Can you work these out from the drawing? Everything is in mm from the part's minimum corner. Coordinates: 2 decimals unless noted, no trailing zeros. Write each loop counter-clockwise with the first axis right and the second up, starting at its lowest first coordinate (ties: lowest second). Pieces come first, ordered by that corner, then holes. Notation, with made-up numbers: M -18.5,65.5 L 18.5,65.5 A30 ccw 18.5,95.5 Z; hole C 11.5,32.25 d11. An arc over 180 degrees is marked long. Answer as a JSON object with one key per item and string values. Group by question number.
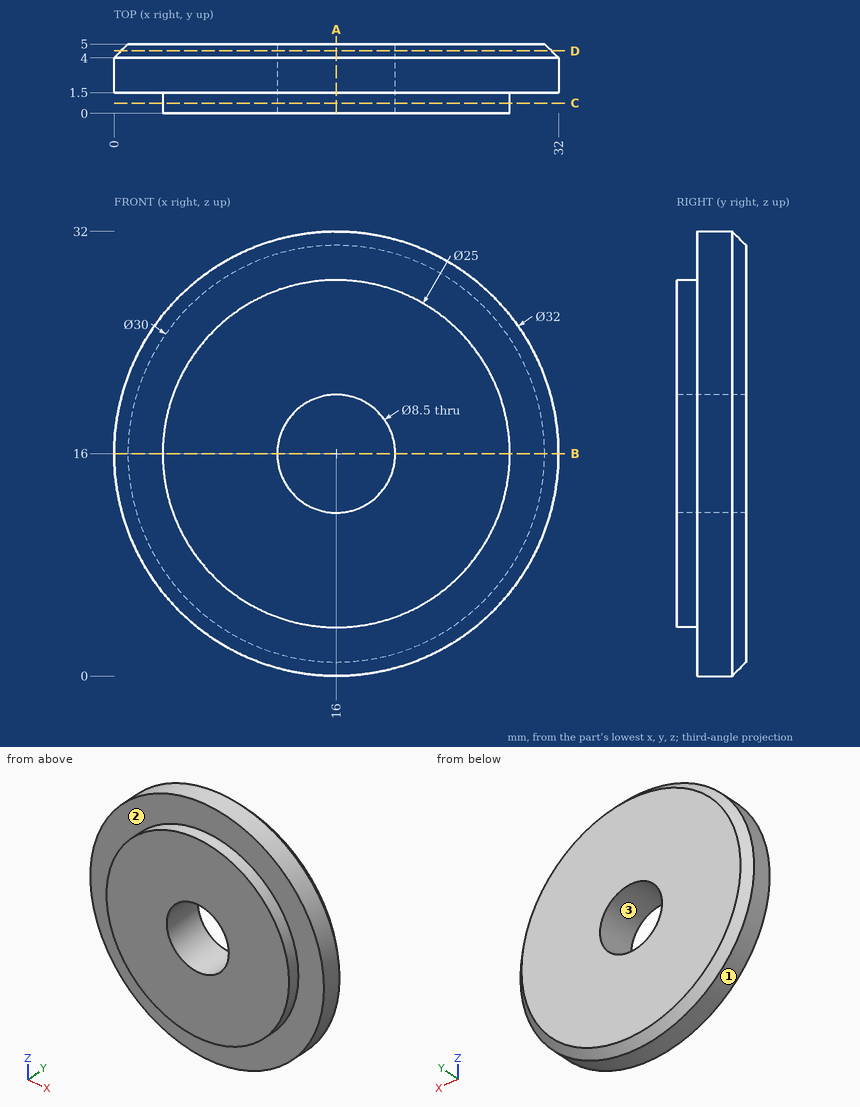
Q1. If we section it at A-A on x = 16: List the corners of the cut face in (y, z) for me.
Q2. Please list where these lines run through material, in increasing order: L1, parallel to Z at x = 16, y = 2.25; L2, parallel to Z at x = 16, y = 1.25; L3, parallel to X at y = 2.8, z = 4.
Q3. Will these pins go through, and if not, where does the flat tip stop? pin 1 (2 mm diameter, centred on y = 2.5, z = 21, fed in from -X); pin 2 (7 mm diameter, centred on x = 16, z = 16, fed in from -Y); pin 3 (3 mm diameter, centred on y = 4, z = 13.5, fed in from +X); pin 4 (2 mm diameter, centred on x = 8.5, y = 3, fed in from +Z).
Q4. If we section it at D-D on y = 4.5: List the corners of the cut face in (x, z) for me, and give its area (3 significant figures).
Q5. If we section it at C-C on y = 0.75: List the corners of the cut face in (x, z) for me, and give its area (3 significant figures).
Q6. If we section it at B-B on z = 16: List the corners of the cut face in (x, y) for me, and give its area (3 significant figures).
Q7. We'd pull the mould along Z, two halves only. Please class the marked faces 1, 2 and 3: pulls with the +Z half, pulls with the -Z half, needs draft (parallel to the pull), parting line crosses it, or undercut.
Reply:
{
 "1": {"outline": "M 0,3.5 L 1.5,3.5 L 1.5,0 L 4,0 L 5,1 L 5,11.75 L 0,11.75 Z; M 0,20.25 L 5,20.25 L 5,31 L 4,32 L 1.5,32 L 1.5,28.5 L 0,28.5 Z"},
 "2": {"L1": "0 to 11.75, 20.25 to 32", "L2": "3.5 to 11.75, 20.25 to 28.5", "L3": "5.42 to 26.58"},
 "3": {"pin 1": "x = 0.51", "pin 2": "through", "pin 3": "x = 31.97", "pin 4": "z = 30.62"},
 "4": {"outline": "C 16,16 d31; hole C 16,16 d8.5", "area": "698 mm^2"},
 "5": {"outline": "C 16,16 d25; hole C 16,16 d8.5", "area": "434 mm^2"},
 "6": {"outline": "M 0,1.5 L 3.5,1.5 L 3.5,0 L 11.75,0 L 11.75,5 L 1,5 L 0,4 Z; M 20.25,0 L 28.5,0 L 28.5,1.5 L 32,1.5 L 32,4 L 31,5 L 20.25,5 Z", "area": "106 mm^2"},
 "7": {"face 1": "parting line crosses it", "face 2": "needs draft", "face 3": "undercut"}
}
